Answer from the drawing. Dimensions are ordinates in mm from the lowest x, y and z of the part. A direction names the side the tool comes from. Coordinates: 2 decimals unless noted, no trailing zeros. Loops run counter-clockwise (first coordinate to the right, second up) from the corner with the lowest first, then second, coordinate; pieces in that order, holes last. Notation, with made-up numbers: (45, 33.25) - (95, 33.25) arc R26 ccw to (95, 60.25) - close; hole circle Ø7 at (-23.75, 44.5). An arc over 180 degrees is marked (long way). Use one line per item in the form item = value. Start each with the question number.
1) A cutting plane is placed at C-C (x = 33). Give the vertices of the cut face in (y, z) (3 decimals), and give its area (3 significant figures).
2) Each of these flat-tipped pins is pushed along its axis until it touches: P1, Ø8, axis at y = 39.5, z = 112, coming from the +X side (3 decimals); P2, Ø1.5, axis at x = 35, y = 74, coming from the +Z side (3 decimals); P3, Ø8, axis at y = 52, z = 220, coming from the -X side. Where does it stop, or does it pass through?
3) Consider line 1 (X direction, y = 100, z = 347.5) (3 decimals). Determine where the line is inside the solid, lowest interval first.
4) A cutting plane is placed at A-A (y = 53.5). Give the vertices of the cut face in (x, z) (3 decimals).
5) A cutting plane is placed at B-B (z = 91). Give the vertices of the cut face in (x, y) (3 decimals).
6) Which of the six approach directions +Z, -Z, +X, -X, +Y, -Y give full straight-line access (tool end or side, diameter ignored) to the marked faces 1 and 2?
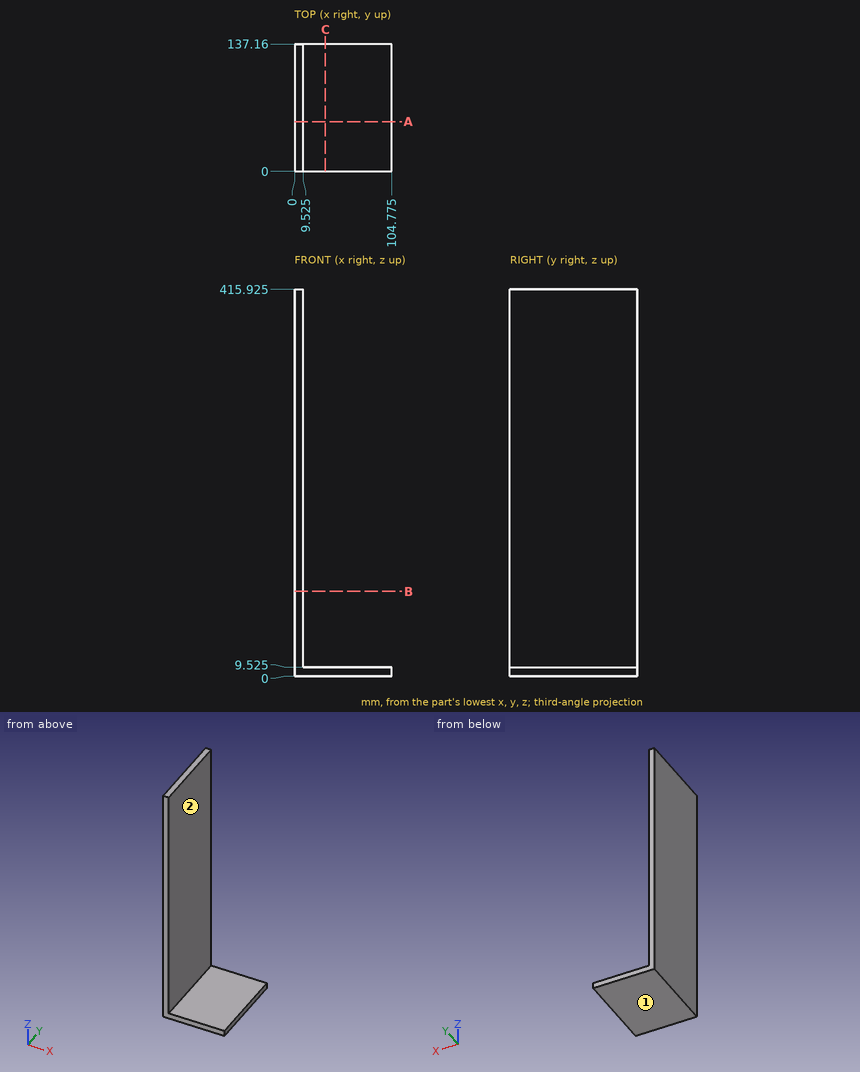
Found:
q1.outline = (0, 0) - (137.16, 0) - (137.16, 9.525) - (0, 9.525) - close
q1.area = 1,310 mm^2
q2.P1 = 9.525
q2.P2 = 9.525
q2.P3 = 0
q3.line_1 = 0 to 9.525
q4.outline = (0, 0) - (104.775, 0) - (104.775, 9.525) - (9.525, 9.525) - (9.525, 415.925) - (0, 415.925) - close
q5.outline = (0, 0) - (9.525, 0) - (9.525, 137.16) - (0, 137.16) - close
q6.face_1 = -Z, +X, -X, +Y, -Y
q6.face_2 = +Z, +X, +Y, -Y
